```python
from build123d import *

# Parameters (mm, degrees)
SKETCH_1_R          = 4.2
EXTRUDE_1_DEPTH     = 4.84
SKETCH_2_R          = 2.5
EXTRUDE_2_DEPTH     = 30
CUT_EXTRUDE_1_DEPTH = 3.4


with BuildPart() as part:
    # 草图1 → 凸台-拉伸1 (new body)
    with BuildSketch(Plane(origin=(0, 0, 0), x_dir=(1, 0, 0), z_dir=(0, 1, 0))):
        Circle(SKETCH_1_R)
    extrude(amount=EXTRUDE_1_DEPTH)

    # 草图2 → 凸台-拉伸2 (add)
    with BuildSketch(Plane(origin=(0, 4.84, 0), x_dir=(1, 0, 0), z_dir=(0, 1, 0))):
        Circle(SKETCH_2_R)
    extrude(amount=EXTRUDE_2_DEPTH)

    # 草图3 → 切除-拉伸1 (cut)
    with BuildSketch(Plane.XZ):
        Polygon((2.3, 0), (1.15, 1.991858429), (-1.15, 1.991858429), (-2.3, 0), (-1.15, -1.991858429), (1.15, -1.991858429), align=None)
    extrude(amount=-CUT_EXTRUDE_1_DEPTH, mode=Mode.SUBTRACT)


solid = part.part
```
For this review, take the finished solid that the model builds, in its own axes (mm). A direction names the side the tool comes from. Coordinates: 2 decimals unless noted, no trailing zeros. Write each loop counter-clockwise with the first axis right and the second up, starting at its lowest first coordinate (ties: lowest second). Pieces come first, ordered by that corner, then holes. Notation, with made-up numbers: (-5.75, -22.75) -> (13.25, -22.75) arc R12 ccw to (13.25, -15.75) -> close; hole circle Ø5 at (83, 18.5). An arc over 180 degrees is marked (long way). Put each result on its own line as item: value.
Q1. Take a section at A-A, the plane x = 0. State the section outline as (y, z) points, then the cut area to 3 significant figures.
From the geometry:
outline: (0, -4.2) -> (4.84, -4.2) -> (4.84, -2.5) -> (34.84, -2.5) -> (34.84, 2.5) -> (4.84, 2.5) -> (4.84, 4.2) -> (0, 4.2) -> (0, 1.99) -> (3.4, 1.99) -> (3.4, -1.99) -> (0, -1.99) -> close
area: 177 mm2
Q2. Take a section at B-B, the plane z = 1.5. State the section outline as (x, y) points, then the cut area to 3 significant figures.
From the geometry:
outline: (-3.92, 0) -> (-1.43, 0) -> (-1.43, 3.4) -> (1.43, 3.4) -> (1.43, 0) -> (3.92, 0) -> (3.92, 4.84) -> (2, 4.84) -> (2, 34.84) -> (-2, 34.84) -> (-2, 4.84) -> (-3.92, 4.84) -> close
area: 148 mm2
Q3. Take a section at D-D, the plane z = -3. State the section outline as (x, y) points, then the cut area to 3 significant figures.
From the geometry:
outline: (-2.94, 0) -> (2.94, 0) -> (2.94, 4.84) -> (-2.94, 4.84) -> close
area: 28.5 mm2
Q4. Take a section at C-C, the plane y = 21.5. State the section outline as (x, z) points, then the cut area to 3 significant figures.
From the geometry:
outline: circle Ø5 at (0, 0)
area: 19.6 mm2
Q5. Clearance check with flat-ended pins moving along their axes: pin 1 Ø1.5 at (y, z) = (22.5, 0.5) entering from -X; pin 2 Ø5 at (x, y) = (-2.5, 15.5) entering from +Z; pin 3 Ø0.7 at (x, y) = (-0.5, 1.5) entering from +Z. State where each tip first meets the part, or that it passes through.
From the geometry:
pin 1: stops at x = -2.5
pin 2: stops at z = 2.5
pin 3: stops at z = 4.2
Q6. Tool access review of faces 4 (the cylindrical face through (4.006, 2.386, -1.262)), 5 (the flat face through (0, 2, 1.992)): name each direction out of +Z, -Z, +X, -X, +Y, -Y from which nothing blocks a thin tool from reaching the whole face with its end or side.
From the geometry:
face 4: +Y, -Y
face 5: -Y
Q7. Wall thickness on L1, parallel to Y at x = 3.5, z = -1; L2, parallel to Y at x = 0.25, z = 1.25; L3, parallel to X at y = 7, z = 0: over which ranges is each line inside the solid? List them lowest first.
From the geometry:
L1: y = 0 to 4.84
L2: y = 3.4 to 34.84
L3: x = -2.5 to 2.5
Q8. The part is to be moulded in two halves that separate along X. For faces 1 (the cylindrical face through (-0.54, 19.63, 2.44)), 2 (the flat face through (0, 3.4, 0)), 3 (the flat face through (2, 4.84, 2)), say which applies: +X half, -X half, draft (parallel to the pull), parting line (faces both ways), or undercut.
From the geometry:
face 1: parting line
face 2: undercut
face 3: draft
